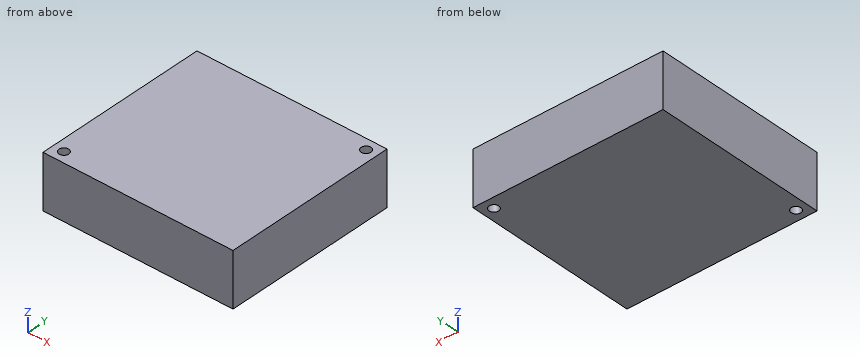
from build123d import *

# Parameters (mm, degrees)
CYLINDER046_R     = 1.2
CYLINDER046_DEPTH = 20
CYLINDER045_R     = 1.2
CYLINDER045_DEPTH = 20
BOX043_W          = 47.1
BOX043_H          = 43.1
BOX043_DEPTH      = 13.4


with BuildPart() as cylinder046:
    # Cylinder046 → Cylinder046 (new body)
    with BuildSketch(Plane(origin=(44.35, 40.35, 0), x_dir=(1, 0, 0), z_dir=(0, 0, 1))):
        Circle(CYLINDER046_R)
    extrude(amount=CYLINDER046_DEPTH)


with BuildPart() as fusion030:
    # Cylinder045 → Cylinder045 (new body)
    with BuildSketch(Plane(origin=(2.75, 2.75, 0), x_dir=(1, 0, 0), z_dir=(0, 0, 1))):
        Circle(CYLINDER045_R)
    extrude(amount=CYLINDER045_DEPTH)

    # Fusion030: union Cylinder046
    add(cylinder046.part)


with BuildPart() as ips7100s:
    # Box043 → Box043 (new body)
    with BuildSketch(Plane.XY):
        with Locations((23.55, 21.55)):
            Rectangle(BOX043_W, BOX043_H)
    extrude(amount=BOX043_DEPTH)

    # Cut012: cut Fusion030
    add(fusion030.part, mode=Mode.SUBTRACT)


with BuildPart() as ips7100s_1:
    # Cut012 placement: moved
    add(ips7100s.part.moved(Location((46.5, 13, 4))))


solid = ips7100s_1.part
Check sheet for the modelled part. Datum: model origin and axes. Units: mm. Round coordinates to 2 decimals unless told otherwise and drop trailing zeros. Loops run counter-clockwise (first coordinate to the right, second up) from the corner with the lowest first, then second, coordinate; pieces in that order, holes last. Notation, with made-up numbers: (18, -32.75) - (39, -32.75) arc R24 ccw to (39, -11.75) - close; hole circle Ø11 at (49, 35). An arc over 180 degrees is marked (long way). Answer as CSV lines item,"result". Start each with the question number.
Item 1: Section check B-B (y = 53.35). Record the boundary of the cut face in (x, z), and give its area (3 significant figures).
Item 2: Section check A-A (x = 90.85). Record the boundary of the cut face in (y, z), and give its area (3 significant figures).
Item 3: Scan lines: line 1 (X direction, y = 53.35, z = 6.75); line 2 (Y direction, x = 49.25, z = 7.75); line 3 (Y direction, x = 90.85, z = 7.5). Record each from-to range of solid material in increasing order. Write a range as [from, to].
Report:
1,outline,"(46.5, 4) - (89.65, 4) - (89.65, 17.4) - (46.5, 17.4) - close; (92.05, 4) - (93.6, 4) - (93.6, 17.4) - (92.05, 17.4) - close"
1,area,"599 mm2"
2,outline,"(13, 4) - (52.15, 4) - (52.15, 17.4) - (13, 17.4) - close; (54.55, 4) - (56.1, 4) - (56.1, 17.4) - (54.55, 17.4) - close"
2,area,"545 mm2"
3,line 1,"x = [46.5, 89.65], [92.05, 93.6]"
3,line 2,"y = [13, 14.55], [16.95, 56.1]"
3,line 3,"y = [13, 52.15], [54.55, 56.1]"
